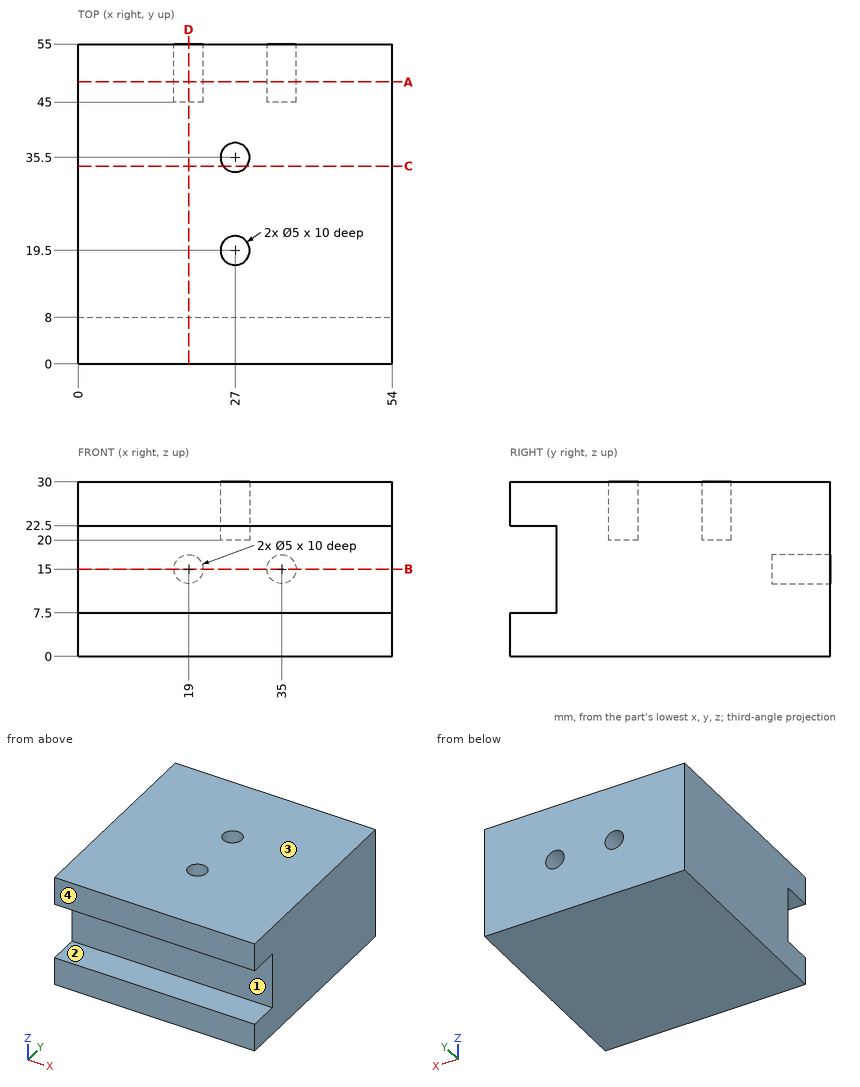
The figure shows three views and two pictorial views of one solid part (mm, origin at its lowest corner). Answer the questions. Round coordinates to 2 decimals unless told otherwise and drop trailing zeros. Loops run counter-clockwise (first coordinate to the right, second up) from the corner with the lowest first, then second, coordinate; pieces in that order, holes last. Notation, with made-up numbers: M 17,-38.75 L 65,-38.75 A26 ccw 65,-21.75 Z; hole C 35.25,77.5 d3. An arc over 180 degrees is marked long. Return JSON: item names as keys, results as strings.
Q1. Find section D-D, the plane x = 19. Determine the outline of the cut face in (y, z).
Results list:
{"outline": "M 0,0 L 55,0 L 55,12.5 L 45,12.5 L 45,17.5 L 55,17.5 L 55,30 L 0,30 L 0,22.5 L 8,22.5 L 8,7.5 L 0,7.5 Z"}
Q2. Find section B-B, the plane z = 15. Determine the outline of the cut face in (x, y), plus the area to 3 significant figures.
Results list:
{"outline": "M 0,8 L 54,8 L 54,55 L 37.5,55 L 37.5,45 L 32.5,45 L 32.5,55 L 21.5,55 L 21.5,45 L 16.5,45 L 16.5,55 L 0,55 Z", "area": "2,440 mm2"}
Q3. The mould has two halves that part along Z. Classify the marked faces 1, 2, 3 and 4: released by +Z, released by -Z, zero draft, split by the parting line, or undercut.
Results list:
{"face 1": "undercut", "face 2": "undercut", "face 3": "released by +Z", "face 4": "zero draft"}
Q4. Find section A-A, the plane y = 48.5. Determine the outline of the cut face in (x, z), plus the area to 3 significant figures.
Results list:
{"outline": "M 0,0 L 54,0 L 54,30 L 0,30 Z; hole C 19,15 d5; hole C 35,15 d5", "area": "1,580 mm2"}
Q5. Each of these flat-tipped pins is pushed along its axis until it touches: pin 1 Ø2.5 at (x, y) = (26.5, 20) entering from +Z; pin 2 Ø1.5 at (x, z) = (35.5, 15.5) entering from +Y; pin 3 Ø1.5 at (x, z) = (15.5, 20) entering from -Y. Where does it stop, or does it pass through?
Results list:
{"pin 1": "stops at z = 20", "pin 2": "stops at y = 45", "pin 3": "stops at y = 8"}
Q6. Find the intervals of material crossed by line 1 along Y through (x, z) = (27, 22.75); line 2 along X through (y, z) = (50.5, 15); line 3 along Y through (x, z) = (28, 24.5), in increasing order. Write a range as from..to.
Results list:
{"line 1": "y = 0..17, 22..33, 38..55", "line 2": "x = 0..16.5, 21.5..32.5, 37.5..54", "line 3": "y = 0..17.21, 21.79..33.21, 37.79..55"}
Q7. Find section C-C, the plane y = 34. Determine the outline of the cut face in (x, z), plus the area to 3 significant figures.
Results list:
{"outline": "M 0,0 L 54,0 L 54,30 L 29,30 L 29,20 L 25,20 L 25,30 L 0,30 Z", "area": "1,580 mm2"}
